Could you check a few things on this model? Use its own coordinates, in mm. Face numbers are marked on the shaded views. A direction names the side the tool comes from. Give positions to 0.01 mm unless a question says otherwise; leave off trailing zeros. Order: outer loops, then holes, each group sorted by start corner. A loop starts at its lowest first (then second) coordinate and runs counter-clockwise, first axis right, second up. Notation, with made-up numbers: (72, -33) -> (127, -33) arc R21 ccw to (127, -21) -> close; hole circle Ø7 at (26, 54.25). An arc over 180 degrees is marked (long way). Write each question's results on one line, items separated by ' | '.
```python
from build123d import *

# Parameters (mm, degrees)
F0_W      = 6
F0_H      = 1.5
F1_DEPTH  = 8
F0_H_2    = 8
F0_R      = 1.5
F2_DEPTH  = 1.5
F4_DEPTH  = 25
F6_DEPTH  = 25
F7_W      = 9.6
F7_H      = 6.5
F8_DEPTH  = 1.5
F9_W      = 6.5
F9_H      = 5
F10_DEPTH = 1.5
F11_W     = 1.5
F11_H     = 19.2
F12_DEPTH = 1.5


# Not quite as in the source:
# - a feature names something its author has since deleted; it is built from what else it names


with BuildPart() as f1:
    # F0 (on Front) → F1 (new body)
    with BuildSketch(Plane.XZ):
        with Locations((4.5, 12.35)):
            Rectangle(F0_W, F0_H)
        with Locations((4.5, 21.85)):
            Rectangle(F0_W, F0_H)
        with Locations((-30.1, 12.35)):
            Rectangle(F0_W, F0_H)
        with Locations((-30.1, 21.85)):
            Rectangle(F0_W, F0_H)
        with BuildLine():
            Line((-27.1, 11.6), (-27.1, -1.5))
            Line((-27.1, -1.5), (1.5, -1.5))
            Line((1.5, -1.5), (1.5, 11.6))
            Line((1.5, 11.6), (1.5, 13.1))
            Line((1.5, 13.1), (1.5, 21.1))
            Line((1.5, 21.1), (1.5, 22.6))
            Line((1.5, 22.6), (1.5, 31.2))
            ThreePointArc((1.5, 31.2), (0.1819805153, 34.3819805153), (-3, 35.7))
            Line((-3, 35.7), (-22.6, 35.7))
            ThreePointArc((-22.6, 35.7), (-25.7819805153, 34.3819805153), (-27.1, 31.2))
            Line((-27.1, 31.2), (-27.1, 22.6))
            Line((-27.1, 22.6), (-27.1, 21.1))
            Line((-27.1, 21.1), (-27.1, 13.1))
            Line((-27.1, 13.1), (-27.1, 11.6))
        make_face()
        with BuildLine():
            ThreePointArc((-25.6, 31.2), (-24.7213203436, 33.3213203436), (-22.6, 34.2))
            Line((-22.6, 34.2), (-3, 34.2))
            ThreePointArc((-3, 34.2), (-0.8786796564, 33.3213203436), (0, 31.2))
            Line((0, 31.2), (0, 0))
            Line((0, 0), (-25.6, 0))
            Line((-25.6, 0), (-25.6, 31.2))
        make_face(mode=Mode.SUBTRACT)
    extrude(amount=F1_DEPTH)

    # F0 (on Front) → F2 (join)
    with BuildSketch(Plane.XZ):
        with Locations((4.5, 17.1)):
            Rectangle(F0_W, F0_H_2)
        with Locations((4.5, 17.1)):
            Circle(F0_R, mode=Mode.SUBTRACT)
        with Locations((-30.1, 17.1)):
            Rectangle(F0_W, F0_H_2)
        with Locations((-30.1, 17.1)):
            Circle(F0_R, mode=Mode.SUBTRACT)
        with BuildLine():
            Line((-3, 34.2), (-22.6, 34.2))
            ThreePointArc((-22.6, 34.2), (-24.7213203436, 33.3213203436), (-25.6, 31.2))
            Line((-25.6, 31.2), (-25.6, 0))
            Line((-25.6, 0), (0, 0))
            Line((0, 0), (0, 31.2))
            ThreePointArc((0, 31.2), (-0.8786796564, 33.3213203436), (-3, 34.2))
        make_face()
    extrude(amount=F2_DEPTH)

    # F3 (on face) → F4 (cut)
    with BuildSketch(Plane(origin=(0, 0, 11.6), x_dir=(1, 0, 0), z_dir=(0, 0, -1))):
        Polygon((7.5, 8), (3, 8), (7.5, 1.5), align=None)
    extrude(amount=-F4_DEPTH, mode=Mode.SUBTRACT)

    # F5 (on face) → F6 (cut)
    with BuildSketch(Plane(origin=(0, 0, 11.6), x_dir=(1, 0, 0), z_dir=(0, 0, -1))):
        Polygon((-33.1, 1.5), (-28.6, 8), (-33.1, 8), align=None)
    extrude(amount=-F6_DEPTH, mode=Mode.SUBTRACT)

    # F7 (on face) → F8 (cut, through all)
    with BuildSketch(Plane(origin=(0, 0, -1.5), x_dir=(1, 0, 0), z_dir=(0, 0, -1))):
        with Locations((-12.8, 4.75)):
            Rectangle(F7_W, F7_H)
    extrude(amount=-F8_DEPTH, mode=Mode.SUBTRACT)

    # F9 (on face) → F10 (cut, through all)
    with BuildSketch(Plane(origin=(-27.1, 0, 0), x_dir=(0, -1, 0), z_dir=(-1, 0, 0))):
        with Locations((4.75, 5)):
            Rectangle(F9_W, F9_H)
    extrude(amount=-F10_DEPTH, mode=Mode.SUBTRACT)

    # F11 (on face) → F12 (cut, through all)
    with BuildSketch(Plane.XZ.offset(1.5)):
        with Locations((-24.35, 17.6)):
            Rectangle(F11_W, F11_H)
        with Locations((-1.25, 17.6)):
            Rectangle(F11_W, F11_H)
    extrude(amount=-F12_DEPTH, mode=Mode.SUBTRACT)


solid = f1.part
```
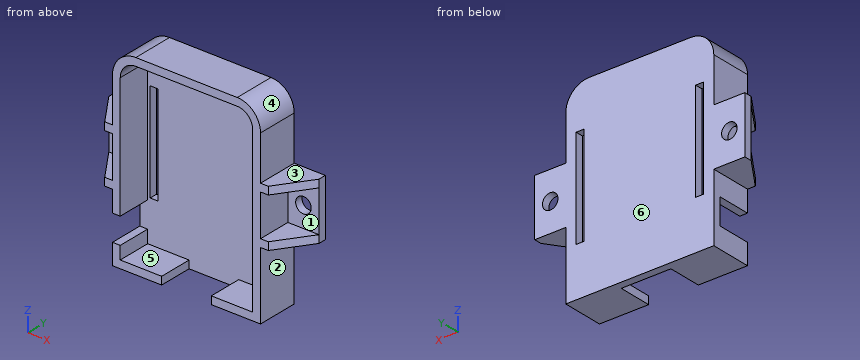
Q1. Suppose I cut it at A-A on z = 10. Please give me the cut outline in (x, y), and give its area (3 significant figures).
Here are the results:
outline: (-27.1, -8) -> (-25.6, -8) -> (-25.6, -1.5) -> (-25.1, -1.5) -> (-25.1, 0) -> (-27.1, 0) -> close; (-23.6, -1.5) -> (-2, -1.5) -> (-2, 0) -> (-23.6, 0) -> close; (-0.5, -1.5) -> (0, -1.5) -> (0, -8) -> (1.5, -8) -> (1.5, 0) -> (-0.5, 0) -> close | area: 57.9 mm²
Q2. For the marked faces 1, 2 and 3, which set-ups out of +Z, -Z, +X, -X, +Y, -Y let a thin tool reach every point of the face, with its end or its side?
Here are the results:
face 1: +X, -Y | face 2: -Z, +X, +Y, -Y | face 3: +Z, +X, +Y, -Y
Q3. I'm going to push flat-ended pins straight in: pin 1 Ø4 at (y, z) = (-2, 25.5) entering from +X; pin 2 Ø4 at (x, z) = (-9, 29.5) entering from -Y; pin 3 Ø1.2 at (x, y) = (-24, -0.5) entering from +Z. Where does each tip first touch, or does it pass through?
Here are the results:
pin 1: stops at x = 1.5 | pin 2: stops at y = -1.5 | pin 3: stops at z = 35.63
Q4. Suppose I cut it at B-B on x = 4. Please give me the cut outline in (y, z).
Here are the results:
outline: (-6.56, 11.6) -> (0, 11.6) -> (0, 15.69) -> (-1.5, 15.69) -> (-1.5, 13.1) -> (-6.56, 13.1) -> close; (-6.56, 21.1) -> (-1.5, 21.1) -> (-1.5, 18.51) -> (0, 18.51) -> (0, 22.6) -> (-6.56, 22.6) -> close
Q5. I need wall thicknesses on line 1 along X through (y, z) = (-7.5, 26.5); line 2 along Z through (x, y) = (-7.5, -6); line 3 along X through (y, z) = (-0.25, 19). Which ranges of each line are inside material? Lowest first, please.
Here are the results:
line 1: x = -27.1 to -25.6, 0 to 1.5 | line 2: z = -1.5 to 0, 34.2 to 35.7 | line 3: x = -33.1 to -25.1, -23.6 to -2, -0.5 to 7.5
Q6. Thinking about a two-plate mould opening in X: for the marked faces 4, 5 and 6, which applies, +X half, -X half, draft (parallel to the pull), parting line (faces both ways), or undercut?
Here are the results:
face 4: +X half | face 5: undercut | face 6: draft
Q7. Suppose I cut it at D-D on z = 17.1. Please give me the cut outline in (x, y), and give its area (3 significant figures).
Here are the results:
outline: (-33.1, -1.5) -> (-31.6, -1.5) -> (-31.6, 0) -> (-33.1, 0) -> close; (-28.6, -1.5) -> (-27.1, -1.5) -> (-27.1, -8) -> (-25.6, -8) -> (-25.6, -1.5) -> (-25.1, -1.5) -> (-25.1, 0) -> (-28.6, 0) -> close; (-23.6, -1.5) -> (-2, -1.5) -> (-2, 0) -> (-23.6, 0) -> close; (-0.5, -1.5) -> (0, -1.5) -> (0, -8) -> (1.5, -8) -> (1.5, -1.5) -> (3, -1.5) -> (3, 0) -> (-0.5, 0) -> close; (6, -1.5) -> (7.5, -1.5) -> (7.5, 0) -> (6, 0) -> close | area: 66.9 mm²
Q8. Suppose I cut it at C-C on y = -1. Please give me the cut outline in (x, z), and give its area (3 significant figures).
Here are the results:
outline: (-33.1, 11.6) -> (-27.1, 11.6) -> (-27.1, -1.5) -> (1.5, -1.5) -> (1.5, 11.6) -> (7.5, 11.6) -> (7.5, 22.6) -> (1.5, 22.6) -> (1.5, 31.2) arc R4.5 ccw to (-3, 35.7) -> (-22.6, 35.7) arc R4.5 ccw to (-27.1, 31.2) -> (-27.1, 22.6) -> (-33.1, 22.6) -> close; hole circle Ø3 at (-30.1, 17.1); hole (-25.1, 8) -> (-23.6, 8) -> (-23.6, 27.2) -> (-25.1, 27.2) -> close; hole (-2, 8) -> (-0.5, 8) -> (-0.5, 27.2) -> (-2, 27.2) -> close; hole circle Ø3 at (4.5, 17.1) | area: 1,120 mm²
